Work out the finished part from the listing and answer in its coordinate system (mm). A direction names the side the tool comes from. Coordinates: 2 decimals unless noted, no trailing zeros. Loops run counter-clockwise (first coordinate to the right, second up) from the corner with the lowest first, then second, coordinate; pieces in that order, holes last. Notation, with made-up numbers: (-13.5, 78.5) -> (12.5, 78.5) arc R9 cw to (12.5, 95.5) -> close; hole circle Ø2 at (-36.75, -19). An arc over 180 degrees is marked (long way). Use a Markdown table: item, result.
from build123d import *

# Parameters (mm, degrees)
ESQUISSE1_W        = 80
ESQUISSE1_H        = 80
BOSS_EXTRU_1_DEPTH = 5


with BuildPart() as part:
    # Esquisse1 → Boss.-Extru.1 (new body)
    with BuildSketch(Plane(origin=(0, 0, 0), x_dir=(1, 0, 0), z_dir=(0, 1, 0))):
        Rectangle(ESQUISSE1_W, ESQUISSE1_H)
    extrude(amount=BOSS_EXTRU_1_DEPTH)

    # Esquisse2 → Révolution2 (revolve)
    with BuildSketch(Plane(origin=(0, 0, 0), x_dir=(0, 0, -1), z_dir=(1, 0, 0)), mode=Mode.PRIVATE) as r_volution2_sk:
        with BuildLine():
            Line((-20, 5), (0, 5))
            Line((0, 5), (0, 25))
            ThreePointArc((0, 25), (-14.142135624, 19.142135624), (-20, 5))
        make_face()
    revolve(r_volution2_sk.sketch.rotate(Axis((0, 5, 0), (0, 1, 0)), 180), axis=Axis((0, 5, 0), (0, 1, 0)))


solid = part.part
Q1. Section B-B on z = -29 is taken. Determine the outline of the cut face in (x, y), and give its area (3 significant figures).
Solved:
| item | result |
|---|---|
| outline | (-40, 0) -> (40, 0) -> (40, 5) -> (-40, 5) -> close |
| area | 400 mm² |
Q2. Given pin 1 Ø2 at (x, y) = (3, 20.5) entering from +Z; pin 2 Ø1.5 at (y, z) = (13, 16) entering from -X; pin 3 Ø24 at (x, z) = (-3.5, -6) entering from +Y; pin 4 Ø3 at (y, z) = (12, -3) entering from +X, each flat-ended and moving along its own axis, determine where each tip first touches the part or whether it passes through.
Solved:
| item | result |
|---|---|
| pin 1 | z = 13.47 |
| pin 2 | x = -10.31 |
| pin 3 | y = 25 |
| pin 4 | x = 19.04 |
Q3. Section D-D on x = 8.5 is taken. Determine the outline of the cut face in (y, z).
Solved:
| item | result |
|---|---|
| outline | (0, -40) -> (5, -40) -> (5, -18.1) arc R18.1 ccw to (5, 18.1) -> (5, 40) -> (0, 40) -> close |
Q4. Section C-C on y = 12.5 is taken. Determine the outline of the cut face in (x, z), and give its area (3 significant figures).
Solved:
| item | result |
|---|---|
| outline | circle Ø37.08 at (0, 0) |
| area | 1,080 mm² |
Q5. Section A-A on x = 25.5 is taken. Determine the outline of the cut face in (y, z).
Solved:
| item | result |
|---|---|
| outline | (0, -40) -> (5, -40) -> (5, 40) -> (0, 40) -> close |
Q6. For faces 1 (the flat face through (-9.4, 5, -18.3)), 2 (the flat face through (40, 2, 1)), determine the directions among +Z, -Z, +X, -X, +Y, -Y from which every point of the face is accessible in a straight line to the end or side of a thin tool.
Solved:
| item | result |
|---|---|
| face 1 | +Y |
| face 2 | +Z, -Z, +X, +Y, -Y |
Q7. Consider line 1 (Y direction, x = -1, z = -28.5); line 2 (Z direction, x = -5.5, y = 7.5); line 3 (X direction, y = 11.5, z = -5.5). Determine where each line is inside the solid, lowest interval first. Write a range as [from, to].
Solved:
| item | result |
|---|---|
| line 1 | [0, 5] |
| line 2 | [-19.07, 19.07] |
| line 3 | [-18.1, 18.1] |
